Input: part model. Units: mm. Frame: model coordinates. Coordinates: 2 decimals unless noted, no trailing zeros. Order: outer loops, then holes, each group sorted by start corner. A loop starts at its lowest first (then second) coordinate and runs counter-clockwise, first axis right, second up. Notation, with made-up numbers: M 0.25,15 L 52.25,15 A6 cw 52.25,21 Z; hole C 73,-2.5 d6. An arc over 180 degrees is marked long. Answer in a Markdown table with one row per item.
from build123d import *

# Parameters (mm, degrees)
SKETCH1_R           = 35
SKETCH1_R_2         = 1
SKETCH1_W           = 22.5
SKETCH1_H           = 12.2
SKETCH1_W_2         = 5
SKETCH1_H_2         = 5
BOSS_EXTRUDE1_DEPTH = 5


with BuildPart() as part:
    # Sketch1 → Boss-Extrude1 (new body)
    with BuildSketch(Plane(origin=(0, 0, 0), x_dir=(1, 0, 0), z_dir=(0, 1, 0))):
        with Locations(Location((0, 0, 0), (0, 0, 270))):
            Circle(SKETCH1_R)
        with Locations(Location((13.75, 0, 0), (0, 0, 270))):
            Circle(SKETCH1_R_2, mode=Mode.SUBTRACT)
        with Locations(Location((-13.75, 0, 0), (0, 0, 270))):
            Circle(SKETCH1_R_2, mode=Mode.SUBTRACT)
        Rectangle(SKETCH1_W, SKETCH1_H, mode=Mode.SUBTRACT)
        with Locations((-20, -20)):
            Rectangle(SKETCH1_W_2, SKETCH1_H_2, mode=Mode.SUBTRACT)
        with Locations((-20, 20)):
            Rectangle(SKETCH1_W_2, SKETCH1_H_2, mode=Mode.SUBTRACT)
        with Locations((20, 20)):
            Rectangle(SKETCH1_W_2, SKETCH1_H_2, mode=Mode.SUBTRACT)
        with Locations((20, -20)):
            Rectangle(SKETCH1_W_2, SKETCH1_H_2, mode=Mode.SUBTRACT)
    extrude(amount=BOSS_EXTRUDE1_DEPTH)


solid = part.part
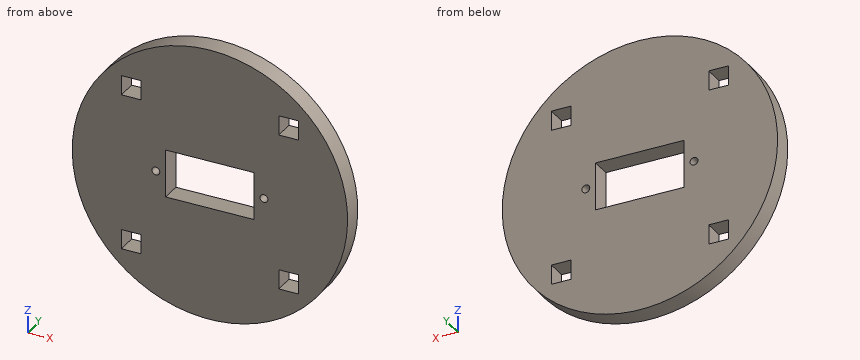
1) Cut plane B-B, the plane z = 0. Output: boundary loops of the cut face in (x, y), and give its area (4 significant figures).
Resolved:
| item | result |
|---|---|
| outline | M -35,0 L -14.75,0 L -14.75,5 L -35,5 Z; M -12.75,0 L -11.25,0 L -11.25,5 L -12.75,5 Z; M 11.25,0 L 12.75,0 L 12.75,5 L 11.25,5 Z; M 14.75,0 L 35,0 L 35,5 L 14.75,5 Z |
| area | 217.5 mm2 |
2) Cut plane A-A, the plane x = 0. Output: boundary loops of the cut face in (y, z).
Resolved:
| item | result |
|---|---|
| outline | M 0,-35 L 5,-35 L 5,-6.1 L 0,-6.1 Z; M 0,6.1 L 5,6.1 L 5,35 L 0,35 Z |
3) Cut plane D-D, the plane x = 13.75. Output: boundary loops of the cut face in (y, z), and give its area (3 significant figures).
Resolved:
| item | result |
|---|---|
| outline | M 0,-32.19 L 5,-32.19 L 5,-1 L 0,-1 Z; M 0,1 L 5,1 L 5,32.19 L 0,32.19 Z |
| area | 312 mm2 |
4) Material intervals for probe 1 along X at (y, z) = (2, 0); probe 2 along Z at (x, y) = (-19, 0.6); probe 3 along Z at (x, y) = (-21.5, 0.3), sorted ascending.
Resolved:
| item | result |
|---|---|
| probe 1 | x = -35 to -14.75, -12.75 to -11.25, 11.25 to 12.75, 14.75 to 35 |
| probe 2 | z = -29.39 to -22.5, -17.5 to 17.5, 22.5 to 29.39 |
| probe 3 | z = -27.62 to -22.5, -17.5 to 17.5, 22.5 to 27.62 |
5) Cut plane C-C, the plane y = 2.5. Output: boundary loops of the cut face in (x, z), and give its area (3 significant figures).
Resolved:
| item | result |
|---|---|
| outline | C 0,0 d70; hole M -22.5,-22.5 L -17.5,-22.5 L -17.5,-17.5 L -22.5,-17.5 Z; hole M -22.5,17.5 L -17.5,17.5 L -17.5,22.5 L -22.5,22.5 Z; hole C -13.75,0 d2; hole M -11.25,-6.1 L 11.25,-6.1 L 11.25,6.1 L -11.25,6.1 Z; hole C 13.75,0 d2; hole M 17.5,-22.5 L 22.5,-22.5 L 22.5,-17.5 L 17.5,-17.5 Z; hole M 17.5,17.5 L 22.5,17.5 L 22.5,22.5 L 17.5,22.5 Z |
| area | 3,470 mm2 |
6) Contact query for flat-ended pins moving along their axis: pin 1 (2.5 mm diameter, centred on x = -19, y = 2, fed in from -Z); pin 2 (1.5 mm diameter, centred on y = 1.5, z = 2.5, fed in from +X); pin 3 (1.5 mm diameter, centred on y = 2.5, z = 20.5, fed in from +X); pin 4 (1.8 mm diameter, centred on x = 13.75, z = 0, fed in from +Y). Output: stop coordinate, or through.
Resolved:
| item | result |
|---|---|
| pin 1 | stops at z = -30.17 |
| pin 2 | stops at x = 34.96 |
| pin 3 | stops at x = 28.9 |
| pin 4 | passes through |
